```python
from build123d import *

# Parameters (mm, degrees)
F0_W     = 25.4
F0_H     = 25.4
F1_DEPTH = 1.411111


with BuildPart() as f1:
    # F0 (on Top) → F1 (new body)
    with BuildSketch(Plane.XY):
        with Locations((12.7, 12.7)):
            Rectangle(F0_W, F0_H)
        Polygon((20.627546, 2.370901), (3.317771, 20.952014), (3.685775, 21.30221), (20.999226, 2.717151), align=None, mode=Mode.SUBTRACT)
    extrude(amount=F1_DEPTH)


solid = f1.part
```
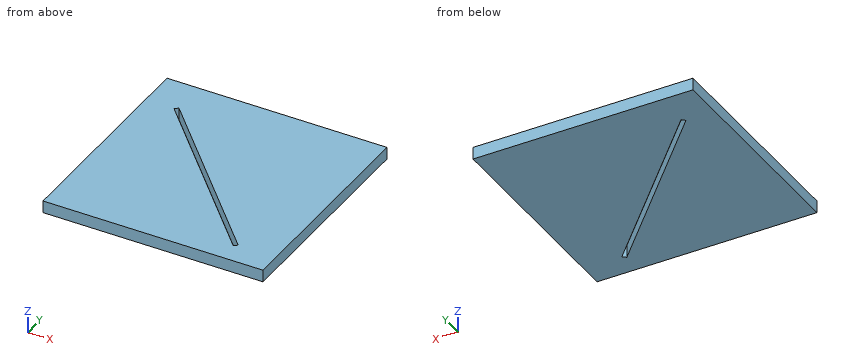
Here's how the part is built. I have some questions about the finished solid (model axes, mm). Give positions to 0.01 mm unless a question says otherwise; leave off trailing zeros. Loops run counter-clockwise (first coordinate to the right, second up) from the corner with the lowest first, then second, coordinate; pieces in that order, holes last. Notation, with made-up numbers: (-13.75, -31) -> (42.25, -31) arc R8 cw to (42.25, -18) -> close; hole circle Ø1 at (19, -23.75). An arc over 180 degrees is marked (long way). Use one line per item in the form item = value. Start each with the question number.
1) Please list where these lines run through material, in increasing order: line 1 along X through (y, z) = (9, 0.15); line 2 along Y through (x, z) = (9.5, 1.15); line 3 along X through (y, z) = (14.75, 0.2).
2) Imagine slicing it at A-A (z = 0.65). Please give me the cut outline in (x, y).
3) Imagine slicing it at B-B (y = 12.75). Please give me the cut outline in (x, z).
4) Imagine slicing it at C-C (x = 12). Please give me the cut outline in (y, z).
Check values:
q1.line_1 = 0 to 14.45, 15.15 to 25.4
q1.line_2 = 0 to 14.32, 15.06 to 25.4
q1.line_3 = 0 to 9.1, 9.79 to 25.4
q2.outline = (0, 0) -> (25.4, 0) -> (25.4, 25.4) -> (0, 25.4) -> close; hole (3.32, 20.95) -> (20.63, 2.37) -> (21, 2.72) -> (3.69, 21.3) -> close
q3.outline = (0, 0) -> (10.96, 0) -> (10.96, 1.41) -> (0, 1.41) -> close; (11.65, 0) -> (25.4, 0) -> (25.4, 1.41) -> (11.65, 1.41) -> close
q4.outline = (0, 0) -> (11.63, 0) -> (11.63, 1.41) -> (0, 1.41) -> close; (12.38, 0) -> (25.4, 0) -> (25.4, 1.41) -> (12.38, 1.41) -> close
